Verification items for the finished model (mm, model axes). Coordinates: 2 decimals unless noted, no trailing zeros. Use one line per item in the form item = value. Start each with the question number.
(1) Gauge pin test, flat ends, axial feed: pin 1 Ø1.5 at (x, z) = (38.5, 1) entering from -Y; pin 2 Ø2.5 at (x, y) = (-14.5, 81.12) entering from -Z; pin 3 Ø1 at (y, z) = (40, 0.5) entering from -X. Record the tip position at first contact, or that the pin passes through.
(2) Material ranges on line 1 (Y direction, x = 25, z = 1.2); line 2 (X direction, y = 61.5, z = 2.1); line 3 (X direction, y = -16, z = 2.85), recorded low to high. Write a range as [from, to].
(3) Sectioned sample at A-A (z = 2.15). Count the separate pieces of the cut face and the enclosed holes in it, and give its area (3 significant figures).
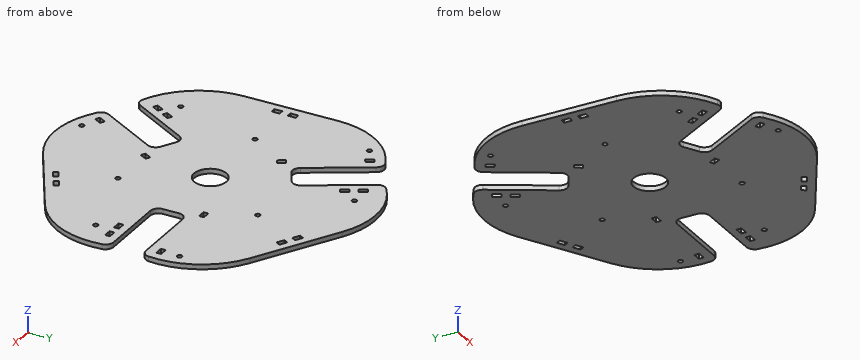
from build123d import *

# Parameters (mm, degrees)
F0_W     = 3
F0_H     = 5
F0_R     = 10
F0_W_2   = 5
F0_H_2   = 3
F1_DEPTH = 3
F2_R     = 1.5
F2_W     = 5
F2_H     = 3
F3_DEPTH = 3


with BuildPart() as f1:
    # F0 (on Top) → F1 (new body)
    with BuildSketch(Plane.XY):
        with BuildLine():
            Line((48.9590259639, 10), (90, 10))
            ThreePointArc((90, 10), (93.331517757, 11.2715969323), (94.96849641, 14.439604226))
            ThreePointArc((94.96849641, 14.439604226), (89.9197428946, 42.5737351708), (70.2835323098, 63.3448321555))
            Line((70.2835323098, 63.3448321555), (45, 77.9422863406))
            Line((45, 77.9422863406), (19.7164676902, 92.5397405257))
            ThreePointArc((19.7164676902, 92.5397405257), (-8.0899352554, 99.1596492339), (-34.9791841247, 89.4649325633))
            ThreePointArc((-34.9791841247, 89.4649325633), (-36.9042695939, 86.4632638174), (-36.3397459622, 82.9422863406))
            Line((-36.3397459622, 82.9422863406), (-15.8192589441, 47.3997602293))
            ThreePointArc((-15.8192589441, 47.3997602293), (-15.3197568316, 43.6056650038), (-17.649385963, 40.5696332104))
            Line((-17.649385963, 40.5696332104), (-26.3096400009, 35.5696332104))
            ThreePointArc((-26.3096400009, 35.5696332104), (-30.1037352264, 35.0701310979), (-33.1397670198, 37.3997602293))
            Line((-33.1397670198, 37.3997602293), (-53.6602540378, 72.9422863406))
            ThreePointArc((-53.6602540378, 72.9422863406), (-56.4272481631, 75.1916668851), (-59.9893122853, 75.0253283373))
            ThreePointArc((-59.9893122853, 75.0253283373), (-81.8298076392, 56.5859140631), (-90, 29.1949083702))
            Line((-90, 29.1949083702), (-90, 0))
            Line((-90, 0), (-90, -29.1949083702))
            ThreePointArc((-90, -29.1949083702), (-81.8298076392, -56.5859140631), (-59.9893122853, -75.0253283373))
            ThreePointArc((-59.9893122853, -75.0253283373), (-56.4272481631, -75.1916668851), (-53.6602540378, -72.9422863406))
            Line((-53.6602540378, -72.9422863406), (-33.1397670198, -37.3997602293))
            ThreePointArc((-33.1397670198, -37.3997602293), (-30.1037352264, -35.0701310979), (-26.3096400009, -35.5696332104))
            Line((-26.3096400009, -35.5696332104), (-17.649385963, -40.5696332104))
            ThreePointArc((-17.649385963, -40.5696332104), (-15.3197568316, -43.6056650038), (-15.8192589441, -47.3997602293))
            Line((-15.8192589441, -47.3997602293), (-36.3397459622, -82.9422863406))
            ThreePointArc((-36.3397459622, -82.9422863406), (-36.9042695939, -86.4632638174), (-34.9791841247, -89.4649325633))
            ThreePointArc((-34.9791841247, -89.4649325633), (-8.0899352554, -99.1596492339), (19.7164676902, -92.5397405257))
            Line((19.7164676902, -92.5397405257), (45, -77.9422863406))
            Line((45, -77.9422863406), (70.2835323098, -63.3448321555))
            ThreePointArc((70.2835323098, -63.3448321555), (89.9197428946, -42.5737351708), (94.96849641, -14.439604226))
            ThreePointArc((94.96849641, -14.439604226), (93.331517757, -11.2715969323), (90, -10))
            Line((90, -10), (48.9590259639, -10))
            ThreePointArc((48.9590259639, -10), (45.423492058, -8.5355339059), (43.9590259639, -5))
            Line((43.9590259639, -5), (43.9590259639, 5))
            ThreePointArc((43.9590259639, 5), (45.423492058, 8.5355339059), (48.9590259639, 10))
        make_face()
        Polygon((-28.1401412901, -86.7401544467), (-30.7382175015, -85.2401544467), (-28.2382175015, -80.9100274278), (-25.6401412901, -82.4100274278), align=None, mode=Mode.SUBTRACT)
        with Locations((-83.5, -5)):
            Rectangle(F0_W, F0_H, mode=Mode.SUBTRACT)
        Polygon((-4.2401412901, -45.3441401458), (-6.8382175015, -43.8441401458), (-4.3382175015, -39.5140131269), (-1.7401412901, -41.0140131269), align=None, mode=Mode.SUBTRACT)
        Polygon((40.3349364905, -74.8621593217), (36.0048094716, -77.3621593217), (34.5048094716, -74.7640831103), (38.8349364905, -72.2640831103), align=None, mode=Mode.SUBTRACT)
        Polygon((48.9951905284, -69.8621593217), (44.6650635095, -72.3621593217), (43.1650635095, -69.7640831103), (47.4951905284, -67.2640831103), align=None, mode=Mode.SUBTRACT)
        with Locations((-83.5, 5)):
            Rectangle(F0_W, F0_H, mode=Mode.SUBTRACT)
        Circle(F0_R, mode=Mode.SUBTRACT)
        Polygon((-37.1491066339, 26.3441401458), (-34.5510304226, 27.8441401458), (-32.0510304226, 23.5140131269), (-34.6491066339, 22.0140131269), align=None, mode=Mode.SUBTRACT)
        Polygon((-61.0491066339, 67.7401544467), (-58.4510304226, 69.2401544467), (-55.9510304226, 64.9100274278), (-58.5491066339, 63.4100274278), align=None, mode=Mode.SUBTRACT)
        with Locations((38.8892479241, 17.5)):
            Rectangle(F0_W_2, F0_H_2, mode=Mode.SUBTRACT)
        with Locations((86.6892479241, 17.5)):
            Rectangle(F0_W_2, F0_H_2, mode=Mode.SUBTRACT)
        Polygon((44.6650635095, 72.3621593217), (48.9951905284, 69.8621593217), (47.4951905284, 67.2640831103), (43.1650635095, 69.7640831103), align=None, mode=Mode.SUBTRACT)
        Polygon((36.0048094716, 77.3621593217), (40.3349364905, 74.8621593217), (38.8349364905, 72.2640831103), (34.5048094716, 74.7640831103), align=None, mode=Mode.SUBTRACT)
    extrude(amount=F1_DEPTH)

    # F2 (on face) → F3 (cut, through all)
    with BuildSketch(Plane.XY.offset(3)):
        with Locations((-50, 0)):
            Circle(F2_R)
        with Locations((25, -43.3012701892)):
            Circle(F2_R)
        with Locations((25, 43.3012701892)):
            Circle(F2_R)
        with Locations((86.6892479241, 29)):
            Circle(F2_R)
        with Locations((-68.4593606718, 60.5750909372)):
            Circle(F2_R)
        with Locations((-18.2298872523, -89.5750909372)):
            Circle(F2_R)
        with Locations((72.5, -16.5)):
            Rectangle(F2_W, F2_H)
        with Locations((82.5, -16.5)):
            Rectangle(F2_W, F2_H)
        Polygon((-24.5096189432, 72.4519052838), (-22.0096189432, 68.1217782649), (-19.4115427319, 69.6217782649), (-21.9115427319, 73.9519052838), align=None)
        Polygon((-29.5096189432, 81.1121593217), (-27.0096189432, 76.7820323028), (-24.4115427319, 78.2820323028), (-26.9115427319, 82.6121593217), align=None)
        Polygon((-50.4903810568, -57.4519052838), (-47.9903810568, -53.1217782649), (-50.5884572681, -51.6217782649), (-53.0884572681, -55.9519052838), align=None)
        Polygon((-55.4903810568, -66.1121593217), (-52.9903810568, -61.7820323028), (-55.5884572681, -60.2820323028), (-58.0884572681, -64.6121593217), align=None)
        with Locations((77.5, -28)):
            Circle(F2_R)
        with Locations((-14.501288694, 81.1169687933)):
            Circle(F2_R)
        with Locations((-62.998711306, -53.1169687933)):
            Circle(F2_R)
    extrude(amount=-F3_DEPTH, mode=Mode.SUBTRACT)


solid = f1.part
Answers below:
q1.pin_1 = -82.13
q1.pin_2 = through
q1.pin_3 = -88.93
q2.line_1 = [-89.49, -44.8], [-41.8, 41.8], [44.8, 89.49]
q2.line_2 = [-78.16, -69.64], [-67.28, -47.05], [-23.96, 73.24]
q2.line_3 = [-90, 70], [75, 80], [85, 95.12]
q3.separate_pieces = 1
q3.enclosed_holes = 28
q3.area = 25,100 mm2
